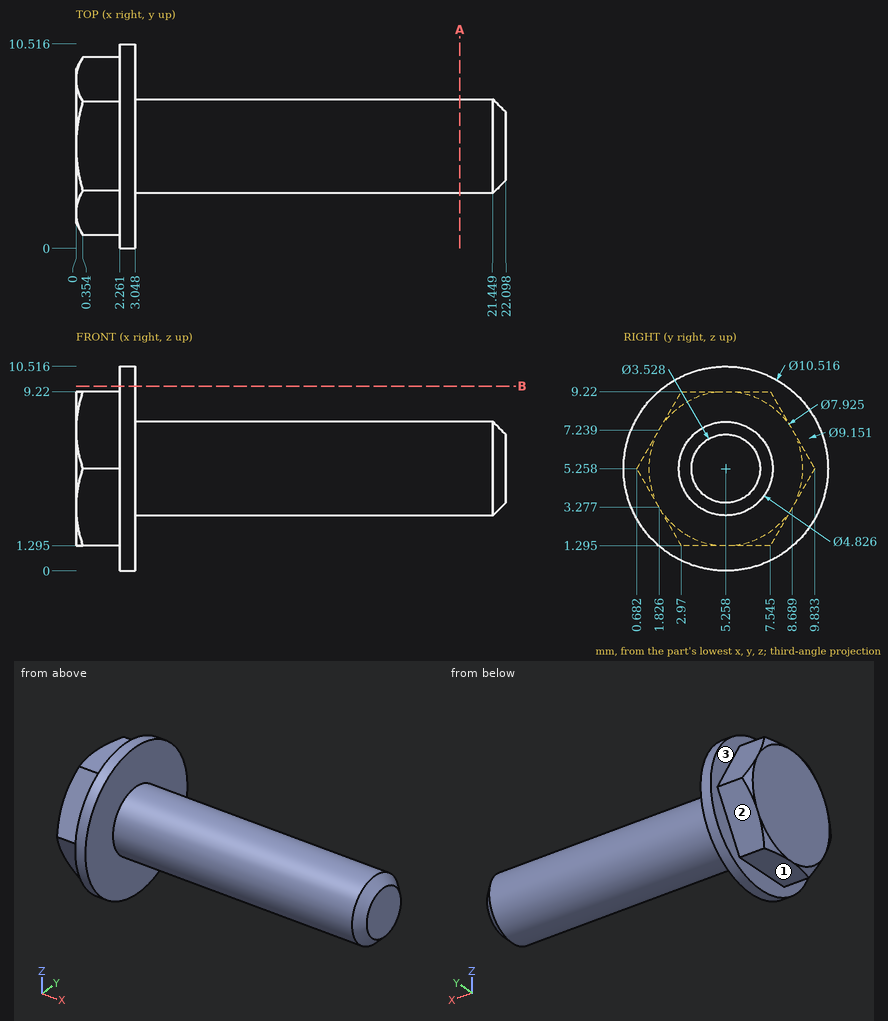
The figure shows three views and two pictorial views of one solid part (mm, origin at its lowest corner). Answer the questions. A direction names the side the tool comes from. Give positions to 0.01 mm unless a question says otherwise; leave off trailing zeros. Order: outer loops, then holes, each group sorted by start corner. A loop starts at its lowest first (then second) coordinate and runs counter-clockwise, first axis right, second up. Notation, with made-up numbers: (24, 29.25) -> (53, 29.25) arc R37 cw to (53, 68.25) -> close; hole circle Ø11 at (-23.5, -5.5). An arc over 180 degrees is marked (long way). One line per item, written item: value.
1) Find the intervals of material crossed by line 1 (X direction, y = 7.5, z = 8.25); line 2 (X direction, y = 9.5, z = 2.5); line 3 (Y direction, x = 15.5, z = 3.25) (1 decimal), in increasing order.
Reported:
line 1: x = 0 to 3.05
line 2: x = 2.26 to 3.05
line 3: y = 3.9 to 6.6
2) Find section B-B, the plane z = 9.5. Determine the outline of the cut face in (x, y).
Reported:
outline: (2.26, 2.15) -> (3.05, 2.15) -> (3.05, 8.36) -> (2.26, 8.36) -> close
3) Find section A-A, the plane x = 19.75. Determine the outline of the cut face in (y, z) (1 decimal).
Reported:
outline: circle Ø4.8 at (5.3, 5.3)
4) Flat-ended cylindrical pins translate along their axes: P1, Ø1, axis at y = 8.5, z = 6.5, coming from the +X side; P2, Ø2, axis at y = 9, z = 4, coming from the -X side; P3, Ø3, axis at x = 17.5, z = 6.5, coming from the -Y side (1 decimal); P4, Ø2.5, axis at x = 0.5, y = 4.5, coming from the +Z side. Find the tip coordinate at first contact, or state that the pin passes through.
Reported:
P1: stops at x = 3.05
P2: stops at x = 0
P3: stops at y = 2.8
P4: stops at z = 9.22
5) A tool of negligible diameter and unlimited length cuts with its end or side. For the marked faces 1, 2 and 3, from which of +Z, -Z, +X, -X, +Y, -Y can it reach the whole face along a straight path? Write none if from no direction.
Reported:
face 1: -Z, -X, +Y, -Y
face 2: -Z, -X, +Y
face 3: -X
